Can you work these out from the model? Positions are in its coordinate system, mm. Face numbers are marked on the shaded views. A direction names the side the tool comes from. Give positions to 0.01 mm unless a question says otherwise; leave off trailing zeros. Write each loop counter-clockwise with the first axis right and the second up, starting at its lowest first coordinate (ties: lowest second). Pieces come first, ordered by that corner, then holes. Notation, with made-up numbers: M 26,73.25 L 30,73.25 A12 cw 30,79.25 Z; hole C 9.5,84.25 d7. An arc over 180 degrees is marked long. Write each question's results on one line, items separated by ' | '.
from build123d import *

# Parameters (mm, degrees)
BASEHEAD_DEPTH   = 15
BEARINGFACESKE_W = 0.8
BEARINGFACESKE_H = 2.784609691
FILLET_2_R       = 0.8


with BuildPart() as part:
    # BaseHeadSke → BaseHead (new body)
    with BuildSketch(Plane(origin=(0, 0, 0), x_dir=(0, 0, -1), z_dir=(1, 0, 0))):
        Polygon((18, 10.392304845), (0, 20.784609691), (-18, 10.392304845), (-18, -10.392304845), (0, -20.784609691), (18, -10.392304845), align=None)
    extrude(amount=BASEHEAD_DEPTH)

    # BodySke → BaseBody (revolve)
    with BuildSketch(Plane.XY):
        Polygon((0, 0), (95, 0), (95, 10.352), (93.352, 12), (0, 12), align=None)
    revolve(axis=Axis((0, 0, 0), (1, 0, 0)))

    # HeadChamferSke → HeadChamfer (revolve, cut)
    with BuildSketch(Plane.XY):
        Polygon((1.607695155, 20.784609691), (0, 20.784609691), (0, 18), align=None)
    revolve(axis=Axis((0, 0, 0), (1, 0, 0)), mode=Mode.SUBTRACT)

    # BearingFaceSke → BearingFace (revolve, cut)
    with BuildSketch(Plane.XY):
        with Locations((14.6, 19.392304845)):
            Rectangle(BEARINGFACESKE_W, BEARINGFACESKE_H)
    revolve(axis=Axis((0, 0, 0), (1, 0, 0)), mode=Mode.SUBTRACT)

    # Fillet 2
    fillet_2_edges = [part.edges().sort_by_distance(p)[0] for p in [
        (15, -12, 0),
    ]]
    fillet(fillet_2_edges, radius=FILLET_2_R)


solid = part.part
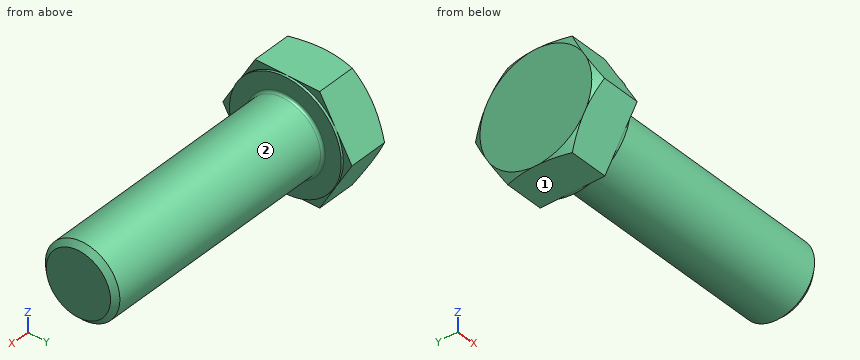
Item 1: I'm going to push flat-ended pins straight in: pin 1 (6 mm diameter, centred on y = -16, z = 6.5, fed in from -X); pin 2 (10 mm diameter, centred on y = -9.5, z = 12.5, fed in from +X); pin 3 (5.5 mm diameter, centred on y = -18, z = 3, fed in from +X); pin 4 (3 mm diameter, centred on x = 68.5, z = 6, fed in from +Y). Where does each tip first touch, or does it pass through?
Geometry says:
pin 1: stops at x = 0 | pin 2: stops at x = 94.65 | pin 3: stops at x = 15 | pin 4: stops at y = 11.12
Item 2: I want a section at B-B, the plane x = 6.5. Please give me the cut outline in (y, z), and give its area (3 significant figures).
Geometry says:
outline: M -20.78,0 L -10.39,-18 L 10.39,-18 L 20.78,0 L 10.39,18 L -10.39,18 Z | area: 1,120 mm2
Item 3: For the marked faces 1 and 2, which set-ups out of +Z, -Z, +X, -X, +Y, -Y let a thin tool reach every point of the face, with its end or its side?
Geometry says:
face 1: -Z, +X, -X, +Y, -Y | face 2: +X
Item 4: I want a section at A-A, the plane x = 63. Please give me the cut outline in (y, z).
Geometry says:
outline: C 0,0 d24
Item 5: If I drill on line 1 (Y direction, x = 32, z = -6); line 2 (X direction, y = -15, z = 8); line 3 (Y direction, x = 59, z = -0.5), over which ranges is the centre line in solid material (lowest first)? Write a range as from..to.
Geometry says:
line 1: y = -10.39..10.39 | line 2: x = 0..15 | line 3: y = -11.99..11.99
